Could you check a few things on this model? Use its own coordinates, in mm. Face numbers are marked on the shaded views. A direction names the side the tool comes from. Round coordinates to 2 decimals unless told otherwise and drop trailing zeros. Loops run counter-clockwise (first coordinate to the right, second up) from the corner with the lowest first, then second, coordinate; pieces in that order, holes last. Notation, with made-up numbers: (60.25, -16.5) - (89.25, -16.5) arc R10 ccw to (89.25, -8.5) - close; hole circle Ø7 at (-38.5, 17). An arc over 180 degrees is marked (long way). Answer as CSV lines item,"result". Start each with the question number.
1) Suppose I cut it at D-D, the plane x = -91.75. Count the separate pieces of the cut face and the enclosed holes in it, then the cut area to 3 significant figures.
2) We'd pull the mould along Y, two halves only. Please class the marked faces 1, 2 and 3: pulls with the +Y half, pulls with the -Y half, needs draft (parallel to the pull), parting line crosses it, or undercut.
3) Suppose I cut it at C-C, the plane y = 26. Write out the boundary of the cut face in (x, z), then the cut area to 3 significant figures.
4) Suppose I cut it at A-A, the plane y = 45.5. Write out the boundary of the cut face in (x, z).
5) Suppose I cut it at B-B, the plane z = 4.75. Write out the boundary of the cut face in (x, y).
6) Which directions (+Z, -Z, +X, -X, +Y, -Y) give clear straight access to the entire face, cutting with the end or side of a thin tool? Please do the marked faces 4, 5 and 6.
7) I'm going to push flat-ended pins straight in: pin 1 Ø4 at (x, y) = (-92.5, 107.5) entering from -Z; pin 2 Ø7.5 at (x, z) = (-94, 15.5) entering from +Y; pin 3 Ø0.7 at (x, z) = (-91, 20.5) entering from -Y. Where does each tip first touch, or does it pass through?
8) Please list where these lines run through material, in increasing order: line 1 along Y through (x, z) = (-91.75, 21.1); line 2 along Y through (x, z) = (-92.5, 1.05); line 3 along X through (y, z) = (48.5, 3.5).
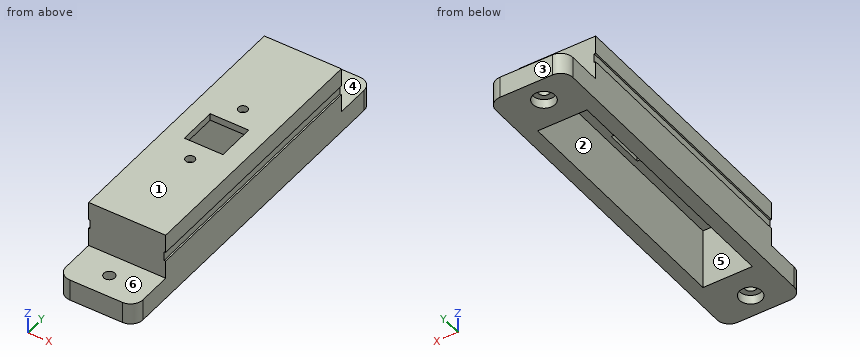
```python
from build123d import *

# Parameters (mm, degrees)
SKETCH019_W     = 25
SKETCH019_H     = 115
PAD002_DEPTH    = 7
SKETCH020_W     = 25
SKETCH020_H     = 85
PAD003_DEPTH    = 15
SKETCH021_W     = 12.5
SKETCH021_H     = 12.5
POCKET017_DEPTH = 22.001
SKETCH022_R     = 1.5
POCKET018_DEPTH = 22.001
SKETCH023_W     = 16
SKETCH023_H     = 80
POCKET019_DEPTH = 19.75
SKETCH024_W     = 1
SKETCH024_H     = 3
POCKET020_DEPTH = 100.001
SKETCH025_R     = 1.8
POCKET021_DEPTH = 22.001
SKETCH026_R     = 3.6
POCKET022_DEPTH = 3
FILLET004_R     = 4


with BuildPart() as part:
    # Sketch019 → Pad002 (new body)
    with BuildSketch(Plane.XY):
        with Locations((-91.75, 57.5)):
            Rectangle(SKETCH019_W, SKETCH019_H)
    extrude(amount=PAD002_DEPTH)

    # Sketch020 → Pad003 (new body)
    with BuildSketch(Plane.XY.offset(7)):
        with Locations((-91.75, 57.5)):
            Rectangle(SKETCH020_W, SKETCH020_H)
    extrude(amount=PAD003_DEPTH)

    # Sketch021 → Pocket017 (cut, through all)
    with BuildSketch(Plane.XY.offset(22)):
        with Locations((-91.75, 58.25)):
            Rectangle(SKETCH021_W, SKETCH021_H)
    extrude(amount=-POCKET017_DEPTH, mode=Mode.SUBTRACT)

    # Sketch022 → Pocket018 (cut, through all)
    with BuildSketch(Plane.XY.offset(22)):
        with Locations((-91.75, 71)):
            Circle(SKETCH022_R)
        with Locations((-91.75, 45.5)):
            Circle(SKETCH022_R)
    extrude(amount=-POCKET018_DEPTH, mode=Mode.SUBTRACT)

    # Sketch023 → Pocket019 (cut)
    with BuildSketch(Plane(origin=(0, 0, 0), x_dir=(1, 0, 0), z_dir=(0, 0, -1))):
        with Locations((-91.75, -57.5)):
            Rectangle(SKETCH023_W, SKETCH023_H)
    extrude(amount=-POCKET019_DEPTH, mode=Mode.SUBTRACT)

    # Sketch024 → Pocket020 (cut, through all)
    with BuildSketch(Plane.XZ.offset(-15)):
        with Locations((-104.25, 14.5)):
            Rectangle(SKETCH024_W, SKETCH024_H)
        with Locations((-79.25, 14.5)):
            Rectangle(SKETCH024_W, SKETCH024_H)
    extrude(amount=-POCKET020_DEPTH, mode=Mode.SUBTRACT)

    # Sketch025 → Pocket021 (cut, through all)
    with BuildSketch(Plane(origin=(0, 0, 0), x_dir=(1, 0, 0), z_dir=(0, 0, -1))):
        with Locations((-92.5, -107.5)):
            Circle(SKETCH025_R)
        with Locations((-92.5, -7.5)):
            Circle(SKETCH025_R)
    extrude(amount=-POCKET021_DEPTH, mode=Mode.SUBTRACT)

    # Sketch026 → Pocket022 (cut)
    with BuildSketch(Plane(origin=(0, 0, 0), x_dir=(1, 0, 0), z_dir=(0, 0, -1))):
        with Locations((-92.5, -7.5)):
            Circle(SKETCH026_R)
        with Locations((-92.5, -107.5)):
            Circle(SKETCH026_R)
    extrude(amount=-POCKET022_DEPTH, mode=Mode.SUBTRACT)

    # Fillet004
    fillet004_edges = [part.edges().sort_by_distance(p)[0] for p in [
        (-104.25, 115, 3.5),
        (-79.25, 115, 3.5),
        (-79.25, 0, 3.5),
        (-104.25, 0, 3.5),
    ]]
    fillet(fillet004_edges, radius=FILLET004_R)


solid = part.part
```
Filled sheet:
1,separate pieces,"6"
1,enclosed holes,"0"
1,area,"390 mm²"
2,face 1,"needs draft"
2,face 2,"undercut"
2,face 3,"pulls with the +Y half"
3,outline,"(-104.25, 0) - (-99.75, 0) - (-99.75, 19.75) - (-83.75, 19.75) - (-83.75, 0) - (-79.25, 0) - (-79.25, 13) - (-79.75, 13) - (-79.75, 16) - (-79.25, 16) - (-79.25, 22) - (-104.25, 22) - (-104.25, 16) - (-103.75, 16) - (-103.75, 13) - (-104.25, 13) - close"
3,area,"231 mm²"
4,outline,"(-104.25, 0) - (-99.75, 0) - (-99.75, 19.75) - (-93.25, 19.75) - (-93.25, 22) - (-104.25, 22) - (-104.25, 16) - (-103.75, 16) - (-103.75, 13) - (-104.25, 13) - close; (-90.25, 19.75) - (-83.75, 19.75) - (-83.75, 0) - (-79.25, 0) - (-79.25, 13) - (-79.75, 13) - (-79.75, 16) - (-79.25, 16) - (-79.25, 22) - (-90.25, 22) - close"
5,outline,"(-104.25, 4) arc R4 ccw to (-100.25, 0) - (-83.25, 0) arc R4 ccw to (-79.25, 4) - (-79.25, 111) arc R4 ccw to (-83.25, 115) - (-100.25, 115) arc R4 ccw to (-104.25, 111) - close; hole (-99.75, 17.5) - (-83.75, 17.5) - (-83.75, 97.5) - (-99.75, 97.5) - close; hole circle Ø3.6 at (-92.5, 7.5); hole circle Ø3.6 at (-92.5, 107.5)"
6,face 4,"+Z, +X, -X, +Y"
6,face 5,"-Z"
6,face 6,"+Z, +X, -X, -Y"
7,pin 1,"z = 3"
7,pin 2,"y = 100"
7,pin 3,"y = 15"
8,line 1,"15 to 44, 47 to 52, 64.5 to 69.5, 72.5 to 100"
8,line 2,"0 to 3.9, 11.1 to 17.5, 97.5 to 103.9, 111.1 to 115"
8,line 3,"-104.25 to -99.75, -83.75 to -79.25"
